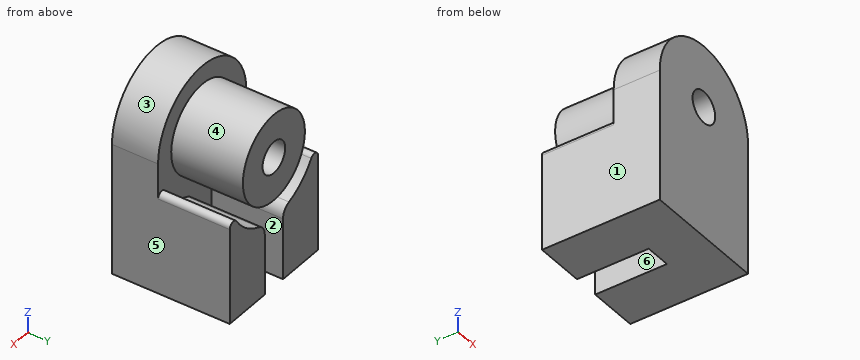
```python
from build123d import *

# Parameters (mm, degrees)
BOSS_EXTRUDE1_DEPTH   = 7
BOSS_EXTRUDE1_2_DEPTH = 7
SKETCH1_R             = 4.25
SKETCH1_R_2           = 1.55
BOSS_EXTRUDE1_3_DEPTH = 7
BOSS_EXTRUDE2_START   = 4.5
SKETCH2_R             = 1.55
BOSS_EXTRUDE2_DEPTH   = 4.5
FILLET1_R             = 0.5
FILLET2_R             = 0.5


with BuildPart() as part:
    # Sketch1 → Boss-Extrude1 (new body)
    with BuildSketch(Plane(origin=(0, 0, 0), x_dir=(1, 0, 0), z_dir=(0, 1, 0))):
        with BuildLine():
            Line((1.25, 12.8585712797929), (1.25, 6.858571279792899))
            ThreePointArc((1.2499999999999998, 6.858571279792899), (1.4758899620338575, 6.141843555941653), (2.0719178082191787, 5.684158389417402))
            ThreePointArc((2.0719178082191805, 5.6841583894174015), (4.956692583756128, 3.468962183440025), (6.049999999999999, -2e-15))
            Line((6.05, 0), (6.05, 9.006664199358159))
            Line((6.05, 9.006664199358159), (6.05, 9.059732997737507))
            Line((6.05, 9.059732997737507), (6.05, 12.8585712797929))
            Line((6.05, 12.8585712797929), (1.25, 12.8585712797929))
        make_face()
    extrude(amount=BOSS_EXTRUDE1_DEPTH)



with BuildPart() as body_2:
    # Sketch1 → Boss-Extrude1 2 (new body)
    with BuildSketch(Plane(origin=(0, 0, 0), x_dir=(1, 0, 0), z_dir=(0, 1, 0))):
        with BuildLine():
            Line((-1.25, 6.858571279792899), (-1.25, 12.8585712797929))
            Line((-1.25, 12.8585712797929), (-6.05, 12.8585712797929))
            Line((-6.05, 12.8585712797929), (-6.05, 9.006664199358159))
            Line((-6.05, 9.006664199358159), (-6.05, 0))
            ThreePointArc((-6.050000000000002, 2.2e-16), (-4.95669258375613, 3.4689621834400257), (-2.0719178082191787, 5.684158389417403))
            ThreePointArc((-2.0719178082191787, 5.684158389417402), (-1.4758899620338577, 6.141843555941653), (-1.25, 6.858571279792899))
        make_face()
    extrude(amount=BOSS_EXTRUDE1_2_DEPTH)


with BuildPart() as body_3:
    # Sketch1 → Boss-Extrude1 3 (new body)
    with BuildSketch(Plane(origin=(0, 0, 0), x_dir=(1, 0, 0), z_dir=(0, 1, 0))):
        with Locations(Location((0, 0, 0), (0, 0, 270))):
            Circle(SKETCH1_R)
        with Locations(Location((0, 0, 0), (0, 0, 270))):
            Circle(SKETCH1_R_2, mode=Mode.SUBTRACT)
    extrude(amount=BOSS_EXTRUDE1_3_DEPTH)


with BuildPart() as part_1:
    add(part.part)

    add(body_2.part)  # Boss-Extrude2 merges body 2

    add(body_3.part)  # Boss-Extrude2 merges body 3
    # Sketch2 → Boss-Extrude2 (add)
    # profile 1 of 4: a face of its own
    with BuildSketch(Plane.XZ.offset(BOSS_EXTRUDE2_START)):
        with BuildLine():
            Line((-6.05, -12.8585712797929), (-1.25, -12.8585712797929))
            Line((-1.25, -12.8585712797929), (-1.2500000000000002, -6.858571279792899))
            ThreePointArc((-1.2500000000000004, -6.858571279792899), (-1.4758899620338575, -6.141843555941654), (-2.071917808219176, -5.684158389417402))
            ThreePointArc((-2.071917808219175, -5.684158389417403), (-4.956692583756129, -3.468962183440026), (-6.05, 5.2e-16))
            Line((-6.05, 7.4e-16), (-6.05, -12.8585712797929))
        make_face()
    # profile 2 of 4: a face of its own
    with BuildSketch(Plane.XZ.offset(BOSS_EXTRUDE2_START)):
        with BuildLine():
            ThreePointArc((2.071917808219175, -5.684158389417404), (1.4758899620338575, -6.141843555941655), (1.25, -6.858571279792899))
            Line((1.25, -6.858571279792899), (1.25, -12.8585712797929))
            Line((1.25, -12.8585712797929), (6.05, -12.8585712797929))
            Line((6.05, -12.8585712797929), (6.05, 0))
            ThreePointArc((6.05, 0), (4.956692583756128, -3.468962183440026), (2.071917808219175, -5.684158389417404))
        make_face()
    # profile 3 of 4: a face of its own
    with BuildSketch(Plane.XZ.offset(BOSS_EXTRUDE2_START)):
        with BuildLine():
            ThreePointArc((6.05, 0), (-4.956692583756127, 3.468962183440027), (2.071917808219173, -5.684158389417404))
            ThreePointArc((2.071917808219173, -5.684158389417404), (4.956692583756128, -3.468962183440026), (6.05, 0))
        make_face()
        with Locations(Location((0, 0, 0), (0, 0, 90))):
            Circle(SKETCH2_R, mode=Mode.SUBTRACT)
    # profile 4 of 4: a face of its own
    with BuildSketch(Plane.XZ.offset(BOSS_EXTRUDE2_START)):
        with BuildLine():
            Line((-1.25, -12.8585712797929), (1.25, -12.8585712797929))
            Line((1.25, -12.8585712797929), (1.2500000000000007, -6.858571279792899))
            ThreePointArc((1.2500000000000002, -6.858571279792899), (1.475889962033857, -6.141843555941656), (2.0719178082191747, -5.684158389417404))
            ThreePointArc((2.0719178082191734, -5.684158389417404), (-7.8e-16, -6.05), (-2.071917808219175, -5.684158389417403))
            ThreePointArc((-2.071917808219176, -5.684158389417402), (-1.4758899620338575, -6.141843555941654), (-1.2500000000000004, -6.858571279792899))
            Line((-1.2500000000000002, -6.858571279792899), (-1.25, -12.8585712797929))
        make_face()
    extrude(amount=-BOSS_EXTRUDE2_DEPTH)

    # Fillet1
    fillet1_edges = [part_1.edges().sort_by_distance(p)[0] for p in [
        (-6.050000000000001, 3.5, -1.1e-16),
    ]]
    fillet(fillet1_edges, radius=FILLET1_R)

    # Fillet2
    fillet2_edges = [part_1.edges().sort_by_distance(p)[0] for p in [
        (6.05, 3.5, 9.4e-16),
    ]]
    fillet(fillet2_edges, radius=FILLET2_R)


solid = part_1.part
```
The model under review builds one solid part; all positions refer to its coordinate system, in mm. Face numbers are marked on the shaded views. A direction names the side the tool comes from. Round coordinates to 2 decimals unless told otherwise and drop trailing zeros. Loops run counter-clockwise (first coordinate to the right, second up) from the corner with the lowest first, then second, coordinate; pieces in that order, holes last. Notation, with made-up numbers: M 69.25,82.5 L 108.25,82.5 A17 cw 108.25,98.5 Z; hole C -21,-22 d2. An arc over 180 degrees is marked long. Put each result on its own line as item: value.
Q1. Mouldability with a two-part tool opening along X and no side actions: class the marked faces 1, 2 and 3 as released by +X, released by -X, zero draft, split by the parting line, or undercut.
Result set:
face 1: released by -X
face 2: undercut
face 3: split by the parting line
Q2. For pin 1 (3 mm diameter, centred on x = -0.5, y = 4.5, fed in from +Z); pin 2 (1.5 mm diameter, centred on x = -2, y = 0, fed in from +Z), all flat-tipped, find the tip position at first contact; note any pin that passes through.
Result set:
pin 1: stops at z = 4.25
pin 2: stops at z = 5.92
Q3. Machinability: for the marked faces 4, 5 and 6, which of the approach directions +Z, -Z, +X, -X, +Y, -Y give a long, thin tool a straight path to every point of the face, cutting with its end or side? Answer none if there is none.
Result set:
face 4: +Y
face 5: +Z, -Z, +X, +Y, -Y
face 6: -Z, +Y
Q4. Consider section B-B, the plane x = 0. Give the boundary of the cut face in (y, z), then the cut area to 3 significant figures.
Result set:
outline: M -4.5,-12.86 L 0,-12.86 L 0,-4.25 L 7,-4.25 L 7,-1.55 L -4.5,-1.55 Z; M -4.5,1.55 L 7,1.55 L 7,4.25 L 0,4.25 L 0,6.05 L -4.5,6.05 Z
area: 109 mm²
Q5. Consider section A-A, the plane y = 2. Give the boundary of the cut face in (x, z), then the cut area to 3 significant figures.
Result set:
outline: M -6.05,-12.86 L -1.25,-12.86 L -1.25,-6.86 A1.25 ccw -2.07,-5.68 A6.05 cw -5.13,-3.21 A0.5 ccw -6.05,-3.48 Z; C 0,0 d8.5; M 1.25,-12.86 L 6.05,-12.86 L 6.05,-3.48 A0.5 ccw 5.13,-3.21 A6.05 cw 2.07,-5.68 A1.25 ccw 1.25,-6.86 Z; hole C 0,0 d3.1
area: 128 mm²
Q6. Consider section D-D, the plane x = -4.5. Give the boundary of the cut face in (y, z).
Result set:
outline: M -4.5,-12.86 L 7,-12.86 L 7,-4.04 L 0,-4.04 L 0,4.04 L -4.5,4.04 Z
Q7. Consider section C-C, the plane z = -10.5. Give the boundary of the cut face in (x, y), then the cut area to 3 significant figures.
Result set:
outline: M -6.05,-4.5 L 6.05,-4.5 L 6.05,7 L 1.25,7 L 1.25,0 L -1.25,0 L -1.25,7 L -6.05,7 Z
area: 122 mm²
Q8. To check wall thickness, follow L1, parallel to Z at x = 0, y = -2.55; L2, parallel to X at y = 5.25, z = -11; L3, parallel to X at y = 3.5, z = 0. State the ranges of each line that lie inside material, in increasing order.
Result set:
L1: z = -12.86 to -1.55, 1.55 to 6.05
L2: x = -6.05 to -1.25, 1.25 to 6.05
L3: x = -4.25 to -1.55, 1.55 to 4.25
